```python
from build123d import *

# Parameters (mm, degrees)
F1_DEPTH  = 400
F2_W      = 60
F2_H      = 60
F3_DEPTH  = 25
F3_FACE_W = 60
F3_FACE_H = 60
F4_DEPTH  = 100


with BuildPart() as f1:
    # F0 (on Top) → F1 (new body)
    with BuildSketch(Plane.XY):
        Polygon((0, 385), (0, 0), (310, 0), (310, 10), (10, 10), (10, 375), (310, 375), (310, 385), align=None)
    extrude(amount=F1_DEPTH)

    # F2 (on face) → F3 (join)
    with BuildSketch(Plane(origin=(0, 385, 0), x_dir=(-1, 0, 0), z_dir=(0, 1, 0))):
        with Locations((-130, 325)):
            Rectangle(F2_W, F2_H)
    extrude(amount=F3_DEPTH)

    # F3_face (on face) → F4 (join)
    with BuildSketch(Plane(origin=(130, 410, 325), x_dir=(-1, 0, 0), z_dir=(0, 1, 0))):
        Rectangle(F3_FACE_W, F3_FACE_H)
    extrude(amount=F4_DEPTH)


solid = f1.part
```
Model file for the job. Use its own axes, mm. A direction names the side the tool comes from. Coordinates: 2 decimals unless noted, no trailing zeros. Loops run counter-clockwise (first coordinate to the right, second up) from the corner with the lowest first, then second, coordinate; pieces in that order, holes last. Notation, with made-up numbers: (79.25, -34) - (105.25, -34) arc R12 ccw to (105.25, -27) - close; hole circle Ø7 at (12, 3.5). An arc over 180 degrees is marked (long way). Write item = value, one per line. Start each with the question number.
Item 1: Pull direction Y, two halves, no side cores. Call faces 1 (the face through (100, 447, 325)), 2 (the face through (130, 510, 325)), 3 (the face through (158, 375, 197)): +Y half, -Y half, draft (parallel to the pull), parting line (faces both ways), or undercut.
Item 2: Saw through at D-D, the plane z = 328. List the corners of the cut face in (x, y).
Item 3: Saw through at A-A, the plane x = 50. List the corners of the cut face in (y, z).
Item 4: 3-axis set-ups, long thin cutter, end or side, ignore diameter. For faces 4 (the face through (160, 447, 325)), 5 (the face through (10, 190, 197)), 6 (the face through (130, 447, 355)), 7 (the face through (130, 447, 295)): which of +Z, -Z, +X, -X, +Y, -Y reach the whole face in a straight line?
Item 5: Drop flat-ended pins along their axis: pin 1 Ø5 at (y, z) = (286.5, 70.5) entering from +X; pin 2 Ø18 at (y, z) = (475.5, 320) entering from -X; pin 3 Ø4 at (x, z) = (242, 277.5) entering from +Y. Give the stop position or say it passes through.
Item 6: Saw through at B-B, the plane z = 238. List the corners of the cut face in (x, y).
Item 7: Wall check: probe 1 along Y at (x, z) = (143, 279); probe 2 along X at (y, z) = (226, 116); probe 3 along Z at (x, y) = (119.5, 458). Give the ranges that are in metal, low to high. Write a range as [from, to].
Item 8: Saw through at C-C, the plane y = 477. List the corners of the cut face in (x, z).
Answers:
q1.face_1 = draft
q1.face_2 = +Y half
q1.face_3 = undercut
q2.outline = (0, 0) - (310, 0) - (310, 10) - (10, 10) - (10, 375) - (310, 375) - (310, 385) - (160, 385) - (160, 510) - (100, 510) - (100, 385) - (0, 385) - close
q3.outline = (0, 0) - (10, 0) - (10, 400) - (0, 400) - close; (375, 0) - (385, 0) - (385, 400) - (375, 400) - close
q4.face_4 = +Z, -Z, +X, +Y
q4.face_5 = +Z, -Z, +X
q4.face_6 = +Z, +X, -X, +Y
q4.face_7 = -Z, +X, -X, +Y
q5.pin_1 = 10
q5.pin_2 = 100
q5.pin_3 = 385
q6.outline = (0, 0) - (310, 0) - (310, 10) - (10, 10) - (10, 375) - (310, 375) - (310, 385) - (0, 385) - close
q7.probe_1 = [0, 10], [375, 385]
q7.probe_2 = [0, 10]
q7.probe_3 = [295, 355]
q8.outline = (100, 295) - (160, 295) - (160, 355) - (100, 355) - close
